from build123d import *

# Parameters (mm, degrees)
BOSS_EXTRUDE1_DEPTH = 1.5
FILLET1_R           = 0.5


with BuildPart() as part:
    # Sketch1 → Boss-Extrude1 (new body)
    with BuildSketch(Plane(origin=(0, 0, 0), x_dir=(1, 0, 0), z_dir=(0, 1, 0))):
        with BuildLine():
            ThreePointArc((0.899416611, 12.4676), (1.956802124, 12.345886985), (3, 12.1346611))
            Line((3, 12.1346611), (3, 12.5))
            ThreePointArc((3, 12.5), (0, 15.5), (-3, 12.5))
            Line((-3, 12.5), (-3, 12.1346611))
            ThreePointArc((-3, 12.1346611), (-1.956802124, 12.345886985), (-0.899416611, 12.4676))
            ThreePointArc((-0.899416611, 12.4676), (-0.016202626, 13.399854141), (0.9, 12.5))
            ThreePointArc((0.9, 12.5), (0.899854141, 12.483797374), (0.899416611, 12.4676))
        make_face()
        with BuildLine():
            ThreePointArc((-3, 6.873863542), (0, 7.5), (3, 6.873863542))
            Line((3, 6.873863542), (3, 12.1346611))
            ThreePointArc((3, 12.1346611), (1.956802124, 12.345886985), (0.899416611, 12.4676))
            ThreePointArc((0.899416611, 12.4676), (0, 11.6), (-0.899416611, 12.4676))
            ThreePointArc((-0.899416611, 12.4676), (-1.956802124, 12.345886985), (-3, 12.1346611))
            Line((-3, 12.1346611), (-3, 6.873863542))
        make_face()
        with BuildLine():
            Line((3, 12.1346611), (3, 6.873863542))
            ThreePointArc((3, 6.873863542), (4.565710718, 5.950150052), (5.863185187, 4.676864277))
            Line((5.863185187, 4.676864277), (10.944725414, 6.038458877))
            ThreePointArc((10.944725414, 6.038458877), (7.609517863, 9.916916754), (3, 12.1346611))
        make_face()
        with BuildLine():
            ThreePointArc((7.5, 0), (7.48822587, -0.420087268), (7.45294045, -0.83885556))
            Line((7.45294045, -0.83885556), (7.772310826, -1.023244132))
            Line((7.772310826, -1.023244132), (12.497639685, 0.24290392))
            ThreePointArc((12.497639685, 0.24290392), (12.43679381, 1.255451998), (12.294047703, 2.259732526))
            ThreePointArc((12.294047703, 2.259732526), (11.108147002, 2.976419019), (11.776823889, 4.190038078))
            ThreePointArc((11.776823889, 4.190038078), (11.39830538, 5.131143582), (10.944725414, 6.038458877))
            Line((10.944725414, 6.038458877), (5.863185187, 4.676864277))
            ThreePointArc((5.863185187, 4.676864277), (7.078979054, 2.477509949), (7.5, 0))
        make_face()
        with BuildLine():
            ThreePointArc((12.294047703, 2.259732526), (12.43679381, 1.255451998), (12.497639685, 0.24290392))
            Line((12.497639685, 0.24290392), (12.850529964, 0.337460585))
            ThreePointArc((12.850529964, 0.337460585), (14.971850307, 4.011695199), (11.297615693, 6.133015543))
            Line((11.297615693, 6.133015543), (10.944725414, 6.038458877))
            ThreePointArc((10.944725414, 6.038458877), (11.39830538, 5.131143582), (11.776823889, 4.190038078))
            ThreePointArc((11.776823889, 4.190038078), (12.666842202, 4.040610319), (13.074072829, 3.235238064))
            ThreePointArc((13.074072829, 3.235238064), (12.855089754, 2.610728206), (12.294047703, 2.259732526))
        make_face()
        with BuildLine():
            Line((12.497639685, 0.24290392), (7.772310826, -1.023244132))
            Line((7.772310826, -1.023244132), (12.008924778, -3.469254338))
            ThreePointArc((12.008924778, -3.469254338), (12.376622312, -1.751918986), (12.5, 0))
            ThreePointArc((12.5, 0), (12.499409907, 0.121457693), (12.497639685, 0.24290392))
        make_face()
        with BuildLine():
            ThreePointArc((7.45294045, -0.83885556), (7.43583646, -0.978946442), (7.416099457, -1.118690681))
            Line((7.416099457, -1.118690681), (7.772310826, -1.023244132))
            Line((7.772310826, -1.023244132), (7.45294045, -0.83885556))
        make_face()
        with BuildLine():
            Line((7.772310826, -1.023244132), (7.416099457, -1.118690681))
            ThreePointArc((7.416099457, -1.118690681), (6.42347811, -3.871553818), (4.45294045, -6.035007983))
            Line((4.45294045, -6.035007983), (9.008924778, -8.665406761))
            ThreePointArc((9.008924778, -8.665406761), (9.713450699, -7.867583842), (10.347550019, -7.012717634))
            ThreePointArc((10.347550019, -7.012717634), (10.045894684, -5.8), (11.24696663, -5.454882366))
            ThreePointArc((11.24696663, -5.454882366), (11.670252823, -4.478303143), (12.008924778, -3.469254338))
            Line((12.008924778, -3.469254338), (7.772310826, -1.023244132))
        make_face()
        with BuildLine():
            ThreePointArc((10.347550019, -7.012717634), (9.713450699, -7.867583842), (9.008924778, -8.665406761))
            Line((9.008924778, -8.665406761), (9.325317547, -8.848076211))
            ThreePointArc((9.325317547, -8.848076211), (13.423393759, -7.75), (12.325317547, -3.651923789))
            Line((12.325317547, -3.651923789), (12.008924778, -3.469254338))
            ThreePointArc((12.008924778, -3.469254338), (11.670252823, -4.478303143), (11.24696663, -5.454882366))
            ThreePointArc((11.24696663, -5.454882366), (11.59651278, -5.786041044), (11.725317547, -6.25))
            ThreePointArc((11.725317547, -6.25), (11.261212732, -7.037397859), (10.347550019, -7.012717634))
        make_face()
        with BuildLine():
            ThreePointArc((4.45294045, -6.035007983), (3.75, -6.495190528), (3, -6.873863542))
            Line((3, -6.873863542), (3, -12.1346611))
            ThreePointArc((3, -12.1346611), (6.25, -10.825317547), (9.008924778, -8.665406761))
            Line((9.008924778, -8.665406761), (4.45294045, -6.035007983))
        make_face()
        with BuildLine():
            Line((3, -12.1346611), (3, -6.873863542))
            ThreePointArc((3, -6.873863542), (0, -7.5), (-3, -6.873863542))
            Line((-3, -6.873863542), (-3, -12.1346611))
            ThreePointArc((-3, -12.1346611), (-2.00620559, -12.337955225), (-0.99919968, -12.46))
            ThreePointArc((-0.99919968, -12.46), (0, -11.5), (0.99919968, -12.46))
            ThreePointArc((0.99919968, -12.46), (2.00620559, -12.337955225), (3, -12.1346611))
        make_face()
        with BuildLine():
            Line((3, -12.5), (3, -12.1346611))
            ThreePointArc((3, -12.1346611), (2.00620559, -12.337955225), (0.99919968, -12.46))
            ThreePointArc((0.99919968, -12.46), (0.9997999, -12.479995997), (1, -12.5))
            ThreePointArc((1, -12.5), (-0.020004003, -13.4997999), (-0.99919968, -12.46))
            ThreePointArc((-0.99919968, -12.46), (-2.00620559, -12.337955225), (-3, -12.1346611))
            Line((-3, -12.1346611), (-3, -12.5))
            ThreePointArc((-3, -12.5), (0, -15.5), (3, -12.5))
        make_face()
        with BuildLine():
            Line((-3, -12.1346611), (-3, -6.873863542))
            ThreePointArc((-3, -6.873863542), (-3.75, -6.495190528), (-4.45294045, -6.035007983))
            Line((-4.45294045, -6.035007983), (-9.008924778, -8.665406761))
            ThreePointArc((-9.008924778, -8.665406761), (-6.25, -10.825317547), (-3, -12.1346611))
        make_face()
        with BuildLine():
            Line((-9.008924778, -8.665406761), (-4.45294045, -6.035007983))
            ThreePointArc((-4.45294045, -6.035007983), (-6.42347811, -3.871553818), (-7.416099457, -1.118690681))
            Line((-7.416099457, -1.118690681), (-7.772310826, -1.023244132))
            Line((-7.772310826, -1.023244132), (-12.008924778, -3.469254338))
            ThreePointArc((-12.008924778, -3.469254338), (-11.670252823, -4.478303143), (-11.24696663, -5.454882366))
            ThreePointArc((-11.24696663, -5.454882366), (-10.361358591, -5.478804767), (-9.925317547, -6.25))
            ThreePointArc((-9.925317547, -6.25), (-10.037919689, -6.685895185), (-10.347550019, -7.012717634))
            ThreePointArc((-10.347550019, -7.012717634), (-9.713450699, -7.867583842), (-9.008924778, -8.665406761))
        make_face()
        with BuildLine():
            Line((-9.325317547, -8.848076211), (-9.008924778, -8.665406761))
            ThreePointArc((-9.008924778, -8.665406761), (-9.713450699, -7.867583842), (-10.347550019, -7.012717634))
            ThreePointArc((-10.347550019, -7.012717634), (-11.604740411, -6.7), (-11.24696663, -5.454882366))
            ThreePointArc((-11.24696663, -5.454882366), (-11.670252823, -4.478303143), (-12.008924778, -3.469254338))
            Line((-12.008924778, -3.469254338), (-12.325317547, -3.651923789))
            ThreePointArc((-12.325317547, -3.651923789), (-13.423393759, -7.75), (-9.325317547, -8.848076211))
        make_face()
        with BuildLine():
            Line((-7.772310826, -1.023244132), (-7.416099457, -1.118690681))
            ThreePointArc((-7.416099457, -1.118690681), (-7.43583646, -0.978946442), (-7.45294045, -0.83885556))
            Line((-7.45294045, -0.83885556), (-7.772310826, -1.023244132))
        make_face()
        with BuildLine():
            Line((-12.008924778, -3.469254338), (-7.772310826, -1.023244132))
            Line((-7.772310826, -1.023244132), (-12.497639685, 0.24290392))
            ThreePointArc((-12.497639685, 0.24290392), (-12.393060767, -1.631577403), (-12.008924778, -3.469254338))
        make_face()
        with BuildLine():
            ThreePointArc((-7.45294045, -0.83885556), (-7.206635264, 2.07711535), (-5.863185187, 4.676864277))
            Line((-5.863185187, 4.676864277), (-10.944725414, 6.038458877))
            ThreePointArc((-10.944725414, 6.038458877), (-11.39830538, 5.131143582), (-11.776823889, 4.190038078))
            ThreePointArc((-11.776823889, 4.190038078), (-11.268700573, 3.828007437), (-11.074072829, 3.235238064))
            ThreePointArc((-11.074072829, 3.235238064), (-11.44956297, 2.454221139), (-12.294047703, 2.259732526))
            ThreePointArc((-12.294047703, 2.259732526), (-12.43679381, 1.255451998), (-12.497639685, 0.24290392))
            Line((-12.497639685, 0.24290392), (-7.772310826, -1.023244132))
            Line((-7.772310826, -1.023244132), (-7.45294045, -0.83885556))
        make_face()
        with BuildLine():
            ThreePointArc((-11.776823889, 4.190038078), (-11.39830538, 5.131143582), (-10.944725414, 6.038458877))
            Line((-10.944725414, 6.038458877), (-11.297615693, 6.133015543))
            ThreePointArc((-11.297615693, 6.133015543), (-14.971850307, 4.011695199), (-12.850529964, 0.337460585))
            Line((-12.850529964, 0.337460585), (-12.497639685, 0.24290392))
            ThreePointArc((-12.497639685, 0.24290392), (-12.43679381, 1.255451998), (-12.294047703, 2.259732526))
            ThreePointArc((-12.294047703, 2.259732526), (-13.039998655, 3.494057109), (-11.776823889, 4.190038078))
        make_face()
        with BuildLine():
            ThreePointArc((-5.863185187, 4.676864277), (-4.565710718, 5.950150052), (-3, 6.873863542))
            Line((-3, 6.873863542), (-3, 12.1346611))
            ThreePointArc((-3, 12.1346611), (-7.609517863, 9.916916754), (-10.944725414, 6.038458877))
            Line((-10.944725414, 6.038458877), (-5.863185187, 4.676864277))
        make_face()
    extrude(amount=BOSS_EXTRUDE1_DEPTH)

    # Fillet1
    fillet1_edges = [part.edges().sort_by_distance(p)[0] for p in [
        (-3, 0.75, 12.1346611),
        (3, 0.75, 12.1346611),
        (9.008924778, 0.75, 8.665406761),
        (12.008924778, 0.75, 3.469254338),
        (12.497639685, 0.75, -0.24290392),
        (10.944725414, 0.75, -6.038458877),
        (3, 0.75, -12.1346611),
        (-3, 0.75, -12.1346611),
        (-10.944725414, 0.75, -6.038458877),
        (-12.497639685, 0.75, -0.24290392),
        (-12.008924778, 0.75, 3.469254338),
        (-9.008924778, 0.75, 8.665406761),
    ]]
    fillet(fillet1_edges, radius=FILLET1_R)


solid = part.part
Could you check a few things on this model? Use its own coordinates, in mm. A direction names the side the tool comes from. Give positions to 0.01 mm unless a question says otherwise; leave off trailing zeros. Order: outer loops, then holes, each group sorted by start corner. A loop starts at its lowest first (then second) coordinate and runs counter-clockwise, first axis right, second up. Notation, with made-up numbers: (-8.75, 51) -> (27.25, 51) arc R27 ccw to (27.25, 77) -> close; hole circle Ø5 at (38, 82). An arc over 180 degrees is marked (long way). Answer in a Markdown table with one row per item. Add a question column.
Item 1: I'm going to push a flat-ended pin straight in: P1, Ø6, axis at x = -7.5, z = -6, coming from the -Y side. Where does the tip first touch, or does it pass through?
Item 2: Imagine slicing it at D-D (y = 1.1). Count the separate pieces of the cut face and the enclosed holes in it, and give its area (3 significant figures).
Item 3: Imagine slicing it at B-B (x = 5.5). List the corners of the cut face in (y, z) for me.
Item 4: Imagine slicing it at A-A (x = 0). List the corners of the cut face in (y, z) for me.
Item 5: We'd pull the mould along Z, two halves only. Please class faces 1 (the cylindrical face through (-0.1, 0.7, 15.5)), 2 (the cylindrical face through (-7.556, 0.739, -9.957)), 3 (the flat face through (-4, 0, 7)), 4 (the cylindrical face through (12.39, 0.74, 1.65)): pulls with the +Z half, pulls with the -Z half, needs draft (parallel to the pull), parting line crosses it, or undercut.
Item 6: Imagine slicing it at C-C (z = -11). List the corners of the cut face in (x, y) for me, and give its area (3 significant figures).
Item 7: Please list where these lines run through material, in increasing order: probe 1 along Z at (x, y) = (11.5, 0.45); probe 2 along Z at (x, y) = (-1.5, 0.8); probe 3 along Z at (x, y) = (11, 0.1).
Item 8: For faces 5 (the cylindrical face through (-12.396, 0.74, 1.611)), 6 (the flat face through (-4, 1.5, 7)), which set-ups out of +Z, -Z, +X, -X, +Y, -Y let a thin tool reach every point of the face, with its end or its side?
Result:
| question | item | result |
|---|---|---|
| 1 | P1 | y = 0 |
| 2 | separate pieces | 1 |
| 2 | enclosed holes | 7 |
| 2 | area | 387 mm2 |
| 3 | outline | (0, -11.22) -> (1.5, -11.22) -> (1.5, -5.1) -> (0, -5.1) -> close; (0, 5.1) -> (1.5, 5.1) -> (1.5, 11.22) -> (0, 11.22) -> close |
| 4 | outline | (0, -15.5) -> (1.5, -15.5) -> (1.5, -13.4) -> (0, -13.4) -> close; (0, -11.6) -> (1.5, -11.6) -> (1.5, -7.5) -> (0, -7.5) -> close; (0, 7.5) -> (1.5, 7.5) -> (1.5, 11.5) -> (0, 11.5) -> close; (0, 13.5) -> (1.5, 13.5) -> (1.5, 15.5) -> (0, 15.5) -> close |
| 5 | face 1 | pulls with the +Z half |
| 5 | face 2 | pulls with the -Z half |
| 5 | face 3 | needs draft |
| 5 | face 4 | undercut |
| 6 | outline | (-5.94, 0) -> (5.94, 0) -> (5.94, 1.5) -> (-5.94, 1.5) -> close |
| 6 | area | 17.8 mm2 |
| 7 | probe 1 | -6.18 to -4.05, -2.42 to 5.65, 6.85 to 9.17 |
| 7 | probe 2 | -15.1 to -7.35, 7.35 to 15.1 |
| 7 | probe 3 | -6.16 to 5.37, 7.13 to 9.24 |
| 8 | face 5 | -X, +Y, -Y |
| 8 | face 6 | +Z, -Z, +X, -X, +Y |
